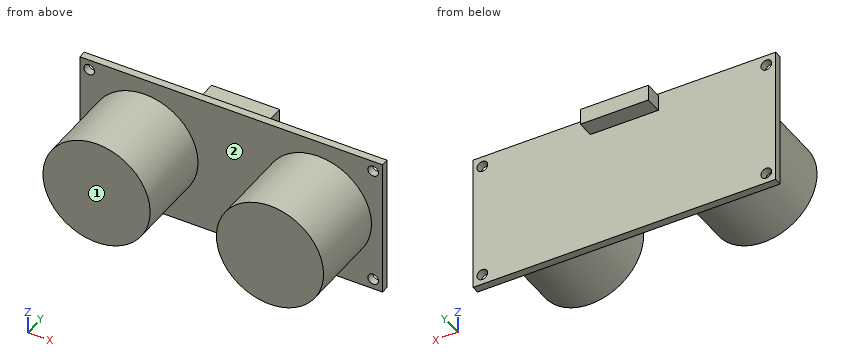
from build123d import *

# Parameters (mm, degrees)
SKETCH1_W           = 22.606
SKETCH1_H           = 10.3251
SKETCH1_R           = 0.8
BOSS_EXTRUDE1_DEPTH = 0.5715
SKETCH3_W           = 5.08
SKETCH3_H           = 2.3876
BOSS_EXTRUDE2_DEPTH = 2.54
SKETCH4_R           = 8.001
BOSS_EXTRUDE3_DEPTH = 12.192


with BuildPart() as part:
    # Sketch1 → Boss-Extrude1 (new, symmetric)
    with BuildSketch(Plane(origin=(0, 0, 0), x_dir=(1, 0, 0), z_dir=(0, 1, 0))):
        with Locations((-11.303, 5.16255)):
            Rectangle(SKETCH1_W, SKETCH1_H)
        with Locations(Location((-21.209, 8.7757, 0), (0, 0, 270))):
            Circle(SKETCH1_R, mode=Mode.SUBTRACT)
    boss_extrude1 = extrude(amount=BOSS_EXTRUDE1_DEPTH, both=True)

    # Mirror1: Boss-Extrude1 across Front Plane
    add(boss_extrude1.mirror(Plane.XY))

    # Sketch3 → Boss-Extrude2 (add)
    with BuildSketch(Plane(origin=(0, 0.5715, 0), x_dir=(1, 0, 0), z_dir=(0, 1, 0))):
        with Locations((-2.54, -8.8773)):
            Rectangle(SKETCH3_W, SKETCH3_H)
    extrude(amount=BOSS_EXTRUDE2_DEPTH)

    # Sketch4 → Boss-Extrude3 (add)
    with BuildSketch(Plane.XZ.offset(0.5715)):
        with Locations(Location((-12.954, 0, 0), (0, 0, 90))):
            Circle(SKETCH4_R)
    extrude(amount=BOSS_EXTRUDE3_DEPTH)

    # Mirror3: part across plane


with BuildPart() as part_1:
    add(part.part)
    add(part.part.mirror(Plane(origin=(0, 0, 0), x_dir=(0, 0, 1), z_dir=(1, 0, 0))))


solid = part_1.part
Work out the finished part from the listing and answer in its coordinate system (mm). Face numbers are marked on the shaded views. A direction names the side the tool comes from. Give positions to 0.01 mm unless a question says otherwise; leave off trailing zeros. Order: outer loops, then holes, each group sorted by start corner. A loop starts at its lowest first (then second) coordinate and runs counter-clockwise, first axis right, second up. Notation, with made-up numbers: (17, -24) -> (63, -24) arc R33 cw to (63, 7) -> close; hole circle Ø6 at (51.5, 84.25). An arc over 180 degrees is marked (long way). Answer as a JSON object with one key per item and string values. Group by question number.
1. Consider line 1 along Y through (x, z) = (-19, -8); line 2 along X through (y, z) = (-1.75, -5.75); line 3 along X through (y, z) = (-11.25, 5). Determine where each line is inside the solid, lowest interval first. Write a range as [from, to].
2. Section B-B on z = 0 is taken. Determine the outline of the cut face in (x, y) (1 decimal).
3. Section C-C on y = -9 is taken. Determine the outline of the cut face in (x, z).
4. Section D-D on x = 10 is taken. Determine the outline of the cut face in (y, z), plus the area to 3 significant figures.
5. Flat-ended cylindrical pins translate along their axes: pin 1 Ø6 at (x, z) = (-11, -3) entering from +Y; pin 2 Ø8 at (x, z) = (-1, 5) entering from -Y; pin 3 Ø2.5 at (y, z) = (2, 9) entering from +X; pin 4 Ø1.3 at (x, z) = (21.21, 8.78) entering from -Y. Find the tip coordinate at first contact, or state that the pin passes through.
6. A tool of negligible diameter and unlimited length cuts with its end or side. For the marked faces 1 and 2, from which of +Z, -Z, +X, -X, +Y, -Y can it reach the whole face along a straight path? Write none if from no direction.
7. Section A-A on x = -1.5 is taken. Determine the outline of the cut face in (y, z), plus the area to 3 significant figures.
Result sheet:
{
 "1": {"line 1": "y = [-0.57, 0.57]", "line 2": "x = [-18.52, -7.39], [7.39, 18.52]", "line 3": "x = [-19.2, -6.71], [6.71, 19.2]"},
 "2": {"outline": "(-22.6, -0.6) -> (-21, -0.6) -> (-21, -12.8) -> (-5, -12.8) -> (-5, -0.6) -> (5, -0.6) -> (5, -12.8) -> (21, -12.8) -> (21, -0.6) -> (22.6, -0.6) -> (22.6, 0.6) -> (-22.6, 0.6) -> close"},
 "3": {"outline": "circle Ø16 at (-12.95, 0); circle Ø16 at (12.95, 0)"},
 "4": {"outline": "(-12.76, -7.44) -> (-0.57, -7.44) -> (-0.57, -10.33) -> (0.57, -10.33) -> (0.57, 10.33) -> (-0.57, 10.33) -> (-0.57, 7.44) -> (-12.76, 7.44) -> close", "area": "205 mm^2"},
 "5": {"pin 1": "stops at y = 0.57", "pin 2": "stops at y = -0.57", "pin 3": "stops at x = 5.08", "pin 4": "passes through"},
 "6": {"face 1": "+Z, -Z, +X, -X, -Y", "face 2": "-Y"},
 "7": {"outline": "(-0.57, -10.33) -> (0.57, -10.33) -> (0.57, 7.68) -> (3.11, 7.68) -> (3.11, 10.07) -> (0.57, 10.07) -> (0.57, 10.33) -> (-0.57, 10.33) -> close", "area": "29.7 mm^2"}
}
